For this review, take the finished solid that the model builds, in its own axes (mm). Coordinates: 2 decimals unless noted, no trailing zeros. Return JSON: item names as keys, results as strings. Group by question number.
Item 1: For line 1 along Y through (x, z) = (4, 0.75); line 2 along X through (y, z) = (4, 0.35); line 3 along Y through (x, z) = (61.5, 2.3), list the stretches that pass through material, from the lowest coordinate up.
Item 2: Insertion check: pin 1 (2.5 mm diameter, centred on x = 61.88, y = 3.12, fed in from -Z); pin 2 (2 mm diameter, centred on x = 55.5, y = 31, fed in from -Z). Each pin has a flat end and moves straight along its axis. Give the tip position at first contact, or say it passes through.
Item 3: Draft analysis for pull direction Y (two halves, no side actions). For faces 1 (the cylindrical face through (0.86, 0.9, 1.27)), 2 (the flat face through (32, 29, 0)), 3 (the cylindrical face through (3.96, 4.43, 1.23)), state which applies: +Y half, -Y half, draft (parallel to the pull), parting line (faces both ways), or undercut.
```python
from build123d import *

# Parameters (mm, degrees)
BASE_SKETCH_W       = 65
BASE_SKETCH_H       = 58
BOSS_EXTRUDE2_DEPTH = 2.5
MOUNTING_HOLES_R    = 1.56250005
MOUNTING_HOLES_R_2  = 1.5625
CUT_EXTRUDE5_DEPTH  = 2.5
FILLET1_R           = 3


with BuildPart() as part:
    # Base Sketch → Boss-Extrude2 (new body)
    with BuildSketch(Plane.XY):
        with Locations((32.5, 29)):
            Rectangle(BASE_SKETCH_W, BASE_SKETCH_H)
    extrude(amount=BOSS_EXTRUDE2_DEPTH)

    # Mounting Holes → Cut-Extrude5 (cut)
    with BuildSketch(Plane.XY):
        with Locations((3.115503651, 54.884496349)):
            Circle(MOUNTING_HOLES_R)
        with Locations((61.884496349, 54.884496349)):
            Circle(MOUNTING_HOLES_R)
        with Locations((61.884496349, 3.115503651)):
            Circle(MOUNTING_HOLES_R)
        with Locations((3.115503651, 3.115503651)):
            Circle(MOUNTING_HOLES_R_2)
    extrude(amount=CUT_EXTRUDE5_DEPTH, mode=Mode.SUBTRACT)

    # Fillet1
    fillet1_edges = [part.edges().sort_by_distance(p)[0] for p in [
        (0, 0, 1.25),
        (0, 58, 1.25),
        (65, 58, 1.25),
        (65, 0, 1.25),
    ]]
    fillet(fillet1_edges, radius=FILLET1_R)


solid = part.part
```
Findings below:
{
 "1": {"line 1": "y = 0 to 1.83, 4.4 to 53.6, 56.17 to 58", "line 2": "x = 0 to 1.83, 4.4 to 60.6, 63.17 to 65", "line 3": "y = 0 to 1.6, 4.63 to 53.37, 56.4 to 58"},
 "2": {"pin 1": "passes through", "pin 2": "stops at z = 0"},
 "3": {"face 1": "-Y half", "face 2": "draft", "face 3": "undercut"}
}
